```python
from build123d import *

# Parameters (mm, degrees)
SKETCH1_W           = 73
SKETCH1_H           = 53
BOSS_EXTRUDE1_DEPTH = 2
SKETCH2_W           = 73
SKETCH2_H           = 53
SKETCH2_W_2         = 70
SKETCH2_H_2         = 50
BOSS_EXTRUDE2_DEPTH = 1.5
CUT_EXTRUDE1_DEPTH  = 4.5


with BuildPart() as part:
    # Sketch1 → Boss-Extrude1 (new body)
    with BuildSketch(Plane(origin=(0, 0, 0), x_dir=(1, 0, 0), z_dir=(0, 1, 0))):
        Rectangle(SKETCH1_W, SKETCH1_H)
    extrude(amount=BOSS_EXTRUDE1_DEPTH)

    # Sketch2 → Boss-Extrude2 (add)
    with BuildSketch(Plane(origin=(0, 2, 0), x_dir=(1, 0, 0), z_dir=(0, 1, 0))):
        Rectangle(SKETCH2_W, SKETCH2_H)
        Rectangle(SKETCH2_W_2, SKETCH2_H_2, mode=Mode.SUBTRACT)
    extrude(amount=BOSS_EXTRUDE2_DEPTH)

    # Sketch3 → Cut-Extrude1 (cut, through all)
    with BuildSketch(Plane.XZ):
        with BuildLine():
            Line((0.6, -4), (0.6, -16))
            ThreePointArc((0.6, -16), (0, -16.6), (-0.6, -16))
            Line((-0.6, -16), (-0.6, -4))
            ThreePointArc((-0.6, -4), (0, -3.4), (0.6, -4))
        make_face()
        with BuildLine():
            Line((3.6, -6.5), (3.6, -13.5))
            ThreePointArc((3.6, -13.5), (3, -14.1), (2.4, -13.5))
            Line((2.4, -13.5), (2.4, -6.5))
            ThreePointArc((2.4, -6.5), (3, -5.9), (3.6, -6.5))
        make_face()
        with BuildLine():
            Line((-2.4, -6.5), (-2.4, -13.5))
            ThreePointArc((-2.4, -13.5), (-3, -14.1), (-3.6, -13.5))
            Line((-3.6, -13.5), (-3.6, -6.5))
            ThreePointArc((-3.6, -6.5), (-3, -5.9), (-2.4, -6.5))
        make_face()
    extrude(amount=-CUT_EXTRUDE1_DEPTH, mode=Mode.SUBTRACT)


solid = part.part
```
Work out the finished part from the listing and answer in its coordinate system (mm). A direction names the side the tool comes from. Give positions to 0.01 mm unless a question says otherwise; leave off trailing zeros. Loops run counter-clockwise (first coordinate to the right, second up) from the corner with the lowest first, then second, coordinate; pieces in that order, holes last. Notation, with made-up numbers: (48, 16.5) -> (92, 16.5) arc R26 cw to (92, 48.5) -> close; hole circle Ø10 at (41.5, 33.5). An arc over 180 degrees is marked (long way). Write item = value, one per line. Start each with the question number.
(1) Find section C-C on x = -21. Give the vertices of the cut face in (y, z).
(2) Find section A-A on y = 2.55. Give the vertices of the cut face in (x, z).
(3) Find section B-B on z = -20. Give the vertices of the cut face in (x, y).
(4) The mould has two halves that part along Z. Classify faces 4 (the flat face through (2.4, 1, -10)), 5 (the flat face through (-1, 2, 26.5)), 6 (the flat face through (-1, 0, 0)): +Z half, -Z half, draft (parallel to the pull), parting line (faces both ways), or undercut.
(5) Find the intervals of material crossed by probe 1 along X at (y, z) = (0.9, -12); probe 2 along X at (y, z) = (2.05, 0); probe 3 along Z at (x, y) = (12, 3.2), in increasing order. Write a range as from..to.
(6) Given pin 1 Ø10 at (x, z) = (-5.5, 13.5) entering from +Y, flat-ended and moving along its own axis, determine where the tip first touches the part or whether it passes through.
(7) Which of the six approach directions +Z, -Z, +X, -X, +Y, -Y give full straight-line access (tool end or side, diameter ignored) to faces 1 (the flat face through (-2.4, 1, -10)), 2 (the flat face through (36.5, 2, 0)), 3 (the flat face through (-35, 3, 0))?
From the geometry:
q1.outline = (0, -26.5) -> (3.5, -26.5) -> (3.5, -25) -> (2, -25) -> (2, 25) -> (3.5, 25) -> (3.5, 26.5) -> (0, 26.5) -> close
q2.outline = (-36.5, -26.5) -> (36.5, -26.5) -> (36.5, 26.5) -> (-36.5, 26.5) -> close; hole (-35, -25) -> (35, -25) -> (35, 25) -> (-35, 25) -> close
q3.outline = (-36.5, 0) -> (36.5, 0) -> (36.5, 3.5) -> (35, 3.5) -> (35, 2) -> (-35, 2) -> (-35, 3.5) -> (-36.5, 3.5) -> close
q4.face_4 = undercut
q4.face_5 = +Z half
q4.face_6 = draft
q5.probe_1 = -36.5..-3.6, -2.4..-0.6, 0.6..2.4, 3.6..36.5
q5.probe_2 = -36.5..-35, 35..36.5
q5.probe_3 = -26.5..-25, 25..26.5
q6.pin_1 = 2
q7.face_1 = +Y, -Y
q7.face_2 = +Z, -Z, +X, +Y, -Y
q7.face_3 = +Y
